```python
from build123d import *

# Parameters (mm, degrees)
F0_R     = 15.875
F1_DEPTH = 31.75
F2_R     = 6.8433299252
F3_DEPTH = 6.35
F4_DEPTH = 6.35
F5_R     = 11.1125
F6_DEPTH = 9.525
F7_R     = 4.7625
F8_DEPTH = 25.4
F9_SIZE2 = 8.89
F9_SIZE  = 31.75


# Not quite as in the source:
# - a fillet or chamfer that OpenCascade refuses, or shapes differently, is made with other operations: its cross-section is extruded or revolved along the edge and cut away or added


with BuildPart() as f1:
    # F0 (on Top) → F1 (new body)
    with BuildSketch(Plane.XY):
        Circle(F0_R)
    extrude(amount=F1_DEPTH)

    # F2 (on face) → F3 (join)
    with BuildSketch(Plane(origin=(0, 0, 0), x_dir=(1, 0, 0), z_dir=(0, 0, -1))):
        Circle(F2_R)
    extrude(amount=F3_DEPTH)

    # F4 (add): a face of the model
    f4_faces = [f1.faces().sort_by_distance(p)[0] for p in [
        (0, 0, 31.75),
    ]]
    extrude(f4_faces, amount=F4_DEPTH)

    # F5 (on face) → F6 (cut)
    with BuildSketch(Plane.XY.offset(38.1)):
        Circle(F5_R)
    extrude(amount=-F6_DEPTH, mode=Mode.SUBTRACT)

    # F7 (on face) → F8 (cut)
    with BuildSketch(Plane.XY.offset(28.575)):
        Circle(F7_R)
    extrude(amount=-F8_DEPTH, mode=Mode.SUBTRACT)

    # F9
    f9_edges = [f1.edges().sort_by_distance(p)[0] for p in [
        (-15.875, 0, 0),
    ]]
    f9_side = f1.faces().sort_by_distance((-15.875, 0, 19.05))[0]
    chamfer(f9_edges, length=F9_SIZE, length2=F9_SIZE2, reference=f9_side)

    # F10: chamfer of 5.08 x 7.62 on 1 edges, made by hand

    # F10_s1 → F10_t2 (revolve, cut)
    with BuildSketch(Plane.XZ):
        Polygon((15.875, 30.48), (10.795, 38.1), (15.875, 38.1), align=None)
    revolve(axis=Axis((0, 0, 38.1), (0, 0, 1)), mode=Mode.SUBTRACT)


solid = f1.part
```
Input: part model. Units: mm. Frame: model coordinates. A direction names the side the tool comes from. Give positions to 0.01 mm unless a question says otherwise; leave off trailing zeros. Loops run counter-clockwise (first coordinate to the right, second up) from the corner with the lowest first, then second, coordinate; pieces in that order, holes last. Notation, with made-up numbers: (71, 73.25) -> (112, 73.25) arc R24 cw to (112, 99.25) -> close; hole circle Ø5 at (-24, 11.5). An arc over 180 degrees is marked (long way). Use a Markdown table: item, result.
Q1. Pull-direction query (Y, two-part tool) for faces 3 (the conical face through (-2.46, -11.06, 37.3)), 4 (the flat face through (0, 0, -6.35)), 5 (the flat face through (0, -5, 28.575)), 6 (the cylindrical face through (-3.78, -2.9, 16.05)); classes: pulls with the +Y half, pulls with the -Y half, needs draft (parallel to the pull), parting line crosses it, or undercut.
Entries:
| item | result |
|---|---|
| face 3 | parting line crosses it |
| face 4 | needs draft |
| face 5 | undercut |
| face 6 | undercut |
Q2. Ray query, probe 1 along Y at (x, z) = (0, 31); probe 2 along Y at (x, z) = (0, 35.5); probe 3 along X at (y, z) = (9.5, 30). Return the intervals inside material, ascending. Write a range as from..to.
Entries:
| item | result |
|---|---|
| probe 1 | y = -15.53..-11.11, 11.11..15.53 |
| probe 2 | y = -12.53..-11.11, 11.11..12.53 |
| probe 3 | x = -12.1..-5.77, 5.77..12.1 |
Q3. Section query C-C, the plane z = 11. Return the cut outline in (x, y) (1 decimal).
Entries:
| item | result |
|---|---|
| outline | circle Ø20.1 at (0, 0); hole circle Ø9.5 at (0, 0) |
Q4. First-contact query: P1, Ø3, axis at x = -2, z = 7, coming from the +Y side; P2, Ø3, axis at y = 4.5, z = -0.5, coming from the -X side; P3, Ø4, axis at y = 2.5, z = 3, coming from the -X side; P4, Ø4, axis at y = 11, z = 1.5, coming from the -X side. Flat tips, straight axial feed; report the tip coordinate or a pass-through.
Entries:
| item | result |
|---|---|
| P1 | stops at y = 9.23 |
| P2 | stops at x = -6.29 |
| P3 | stops at x = -8.17 |
| P4 | passes through |
Q5. Section query D-D, the plane z = -4. Return the cut outline in (x, y), plus the area to 3 significant figures.
Entries:
| item | result |
|---|---|
| outline | circle Ø13.69 at (0, 0) |
| area | 147 mm² |
Q6. Access query for faces 1 (the cylindrical face through (-6.837, -0.301, -3.131)), 2 (the flat face through (0, 0, 3.175)). Directions: +Z, -Z, +X, -X, +Y, -Y. A direction counts if a zero-diameter tool reaches every point of the face in a straight line with its end or side. Return the directions, or none.
Entries:
| item | result |
|---|---|
| face 1 | -Z |
| face 2 | +Z |
